Check sheet for the modelled part. Datum: model origin and axes. Units: mm. Face numbers are marked on the shaded views. Give positions to 0.01 mm unless a question says otherwise; leave off trailing zeros. Order: outer loops, then holes, each group sorted by start corner. A loop starts at its lowest first (then second) coordinate and runs counter-clockwise, first axis right, second up.
Item 1: Sectioned sample at C-C on z = -17.5. Record the boundary of the cut face in (x, y).
Item 2: Sectioned sample at A-A on y = 6.5. Record the boundary of the cut face in (x, z).
Item 3: Sectioned sample at D-D on y = 13.75. Record the boundary of the cut face in (x, z), and give its area (3 significant figures).
Item 4: Gauge pin test, flat ends, axial feed: P1, Ø2, axis at x = -5.5, y = 4.5, coming from the +Z side; P2, Ø7.5, axis at y = 8, z = -15, coming from the +X side; P3, Ø0.8, axis at x = -5.5, z = -25.5, coming from the +Y side; P4, Ø4, axis at y = 1.5, z = -20, coming from the -X side. Record the tip position at first contact, or that the pin passes through.
Item 5: Material ranges on line 1 along X through (y, z) = (12, -23.5); line 2 along Y through (x, z) = (-1, -24.25); line 3 along Z through (x, y) = (-8, 4.75), recorded low to high.
Item 6: Sectioned sample at B-B on x = -5.5. Record the boundary of the cut face in (y, z), and give its area (3 significant figures).
Item 7: Release check for a two-part mould opening along Z. For the marked faces 1, 2 and 3 record: released by +Z, released by -Z, zero draft, split by the parting line, or undercut.
Autodesk Inventor part; units mm, degrees
ref_plane "YZ Plane" through (0, 0, 0) normal (1, 0, 0) x (0, 1, 0)
ref_plane "XZ Plane" through (0, 0, 0) normal (0, 1, 0) x (-1, 0, 0)
ref_plane "XY Plane" through (0, 0, 0) normal (0, 0, 1) x (1, 0, 0)
sketch "Sketch2" plane through (0, 0, 0) normal (0, 1, 0) x (-1, 0, 0)
  line L0 (0, 0) -> (0, -26)
  line L1 (0, -26) -> (11, -26)
  line L2 (11, -26) -> (11, 0)
  line L3 (11, 0) -> (0, 0)
  dimension "d2" = 26
  dimension "d3" = 11
extrude "Extrusion1" add sketch "Sketch2" along normal blind 15
sketch "Sketch3" plane through (-11, 0, 0) normal (0, 0, 1) x (1, 0, 0)
  line L0 (0, 0) -> (11, 0)
  line L1 (11, 0) -> (11, 15)
  line L2 (0, 15) -> (11, 15)
  line L3 (0, 0) -> (0, 15)
  line L4 (11, 15) -> (0, 15)
  circle A0 centre (5.5, 15) radius 4.25
  point P0 (9.75, 15)
  point P1 (1.25, 15)
  dimension "d6" = 8.5
extrude "Extrusion2" cut sketch "Sketch3" against normal blind 32.25 contours L2 A0 picked at (4.2044, 14.0026)
sketch "Sketch4" plane through (0, 0, 0) normal (1, 0, 0) x (0, 0, -1)
  line L0 (0, 0) -> (26, 0)
  line L1 (26, 0) -> (26, 15)
  line L2 (0, 15) -> (26, 15)
  line L3 (0, 0) -> (0, 15)
  line L4 (0, 15) -> (4, 15)
  line L5 (0, 15) -> (26, 15)
  line L6 (26, 15) -> (22, 15)
  line L7 (22, 15) -> (22, 12)
  line L8 (0, 10.75) -> (26, 10.75)
  line L9 (22, 12) -> (4, 12)
  line L10 (4, 12) -> (4, 15)
  line L11 (26, 0) -> (0, 0)
  line L12 (13, 0) -> (13, 3)
  arc A0 (4, 12) -> (22, 12) centre (13, 12) ccw
  dimension "d9" = 4
  dimension "d10" = 4
  dimension "d11" = 3
  dimension "d12" = 3
extrude "Extrusion3" cut sketch "Sketch4" against normal blind 32.25 contours A0 L8 | A0 L9 L8 | L2 L7 L9 L10
sketch "Sketch5" plane through (-11, 0, 0) normal (0, 0, 1) x (1, 0, 0)
  arc A0 (1.25, 15) -> (9.75, 15) centre (5.5, 15) ccw
  line L0 (0, 15) -> (1.25, 15)
  line L1 (0, 0) -> (0, 15)
  line L2 (0, 0) -> (11, 0)
  line L3 (11, 0) -> (11, 15)
  line L4 (9.75, 15) -> (11, 15)
  arc A1 (1.25, 15) -> (9.75, 15) centre (5.5, 15) ccw
  line L5 (5.5, 10.75) -> (7, 10.75)
  line L6 (7, 10.75) -> (4, 10.75)
  line L7 (4, 10.75) -> (4.7672, 11.9025)
  line L8 (4.7672, 11.9025) -> (5.5, 11.9025)
  line L9 (5.5, 11.9025) -> (5.5, 10.75)
  line L10 (7, 10.75) -> (6.2328, 11.9025)
  line L11 (6.2328, 11.9025) -> (5.5, 11.9025)
  arc A2 (1.25, 15) -> (9.75, 15) centre (5.5, 15) ccw
  line L12 (11, 15) -> (9.75, 15)
  line L13 (11, 0) -> (11, 15)
  line L14 (11, 0) -> (0, 0)
  line L15 (0, 0) -> (0, 15)
  line L16 (1.25, 15) -> (0, 15)
  line L17 (5.5, 10.75) -> (4, 10.75)
  line L18 (4, 10.75) -> (4.7672, 11.9025)
  line L19 (6.2328, 11.9025) -> (6.1284, 11.9025)
  line L20 (6.2328, 11.9025) -> (4.7672, 11.9025)
  line L21 (6.2328, 11.9025) -> (7, 10.75)
  line L22 (7, 10.75) -> (4, 10.75)
  arc A3 (1.25, 15) -> (9.75, 15) centre (5.5, 15) ccw
  line L23 (11, 15) -> (9.75, 15)
  line L24 (11, 0) -> (11, 15)
  line L25 (11, 0) -> (0, 0)
  line L26 (0, 0) -> (0, 15)
  line L27 (1.25, 15) -> (0, 15)
  arc A4 (1.25, 15) -> (9.75, 15) centre (5.5, 15) ccw
  line L28 (11, 15) -> (9.75, 15)
  line L29 (11, 0) -> (11, 15)
  line L30 (11, 0) -> (0, 0)
  line L31 (0, 0) -> (0, 15)
  line L32 (1.25, 15) -> (0, 15)
  point P0 (4.1472, 10.9711)
  point P1 (6.8528, 10.9711)
  dimension "d15" = 1.5
  dimension "d16" = 3
extrude "Extrusion4" add sketch "Sketch5" against normal blind 1 contours L7 L8 L9 A0 | L9 L11 L10 A0
sketch "Sketch6" plane through (0, 0, -26) normal (0, 0, -1) x (-1, 0, 0)
  arc A0 (1.25, 15) -> (9.75, 15) centre (5.5, 15) ccw
  line L0 (0, 15) -> (1.25, 15)
  line L1 (0, 0) -> (0, 15)
  line L2 (0, 0) -> (11, 0)
  line L3 (11, 0) -> (11, 15)
  line L4 (9.75, 15) -> (11, 15)
  arc A1 (4.1472, 10.9711) -> (6.8528, 10.9711) centre (5.5, 15) ccw
  line L5 (5.5, 10.75) -> (7, 10.75)
  line L6 (4.7672, 11.9025) -> (6.2328, 11.9025)
  line L7 (7, 10.75) -> (6.2328, 11.9025)
  line L8 (6.2328, 11.9025) -> (4.7672, 11.9025)
  line L9 (4.7672, 11.9025) -> (4, 10.75)
  line L10 (4.7672, 11.9025) -> (4.1472, 10.9711)
  line L11 (4, 10.75) -> (5.5, 10.75)
  point P0 (0, 0)
  point P1 (6.8528, 10.9711)
  dimension "d19" = 1.5
extrude "Extrusion5" add sketch "Sketch6" against normal blind 1 contours L9 L6 L7 A0
sketch "Sketch7" plane through (0, 0, 0) normal (0, -1, 0) x (1, 0, 0)
  line L0 (0, -26) -> (-11, -26)
  line L1 (0, 0) -> (0, -26)
  line L2 (-11, 0) -> (0, 0)
  line L3 (-11, -26) -> (-11, 0)
  circle A0 centre (-5.5, -13) radius 5
  dimension "d22" = 10
extrude "Extrusion6" add sketch "Sketch7" along normal blind 2 contours A0
sketch "Sketch8" plane through (-5.5, -2, -13) normal (0, -1, 0) x (1, 0, 0)
  circle A0 centre (0, 0) radius 6
  point P0 (5.5, 13)
  dimension "d25" = 12
extrude "Extrusion7" add sketch "Sketch8" along normal blind 3.5
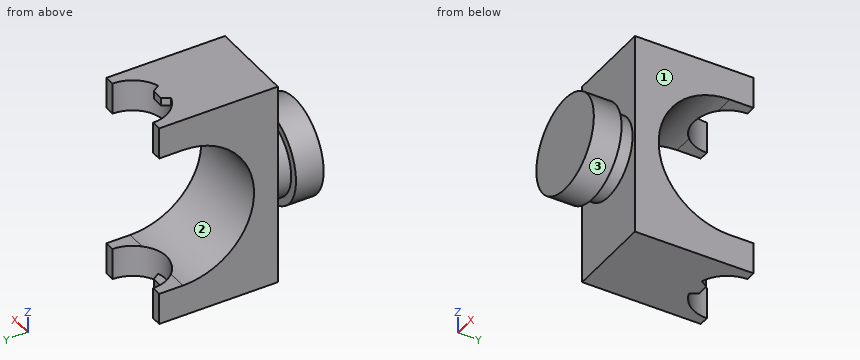
Report:
1. outline: (-11, 0) - (-7.68, 0) - (-7.68, -2) - (-9.47, -2) - (-9.47, -5.5) - (-1.53, -5.5) - (-1.53, -2) - (-3.32, -2) - (-3.32, 0) - (0, 0) - (0, 4.21) - (-11, 4.21) - close
2. outline: (-11, -26) - (0, -26) - (0, -20.12) - (-11, -20.12) - close; (-11, -5.88) - (0, -5.88) - (0, 0) - (-11, 0) - close
3. outline: (-11, -26) - (-9.56, -26) - (-9.56, -22) - (-11, -22) - close; (-11, -4) - (-9.56, -4) - (-9.56, 0) - (-11, 0) - close; (-1.44, -26) - (0, -26) - (0, -22) - (-1.44, -22) - close; (-1.44, -4) - (0, -4) - (0, 0) - (-1.44, 0) - close
3. area: 23.0 mm2
4. P1: stops at z = 0
4. P2: passes through
4. P3: stops at y = 11.9
4. P4: stops at x = -11
5. line 1: x = -11 to -8.51, -2.49 to 0
5. line 2: y = 0 to 15
5. line 3: z = -26 to -18.33, -7.67 to 0
6. outline: (-5.5, -19) - (-2, -19) - (-2, -18) - (0, -18) - (0, -26) - (11.9, -26) - (11.9, -25) - (10.75, -25) - (10.75, -21.91) arc R9 cw to (10.75, -4.09) - (10.75, -1) - (11.9, -1) - (11.9, 0) - (0, 0) - (0, -8) - (-2, -8) - (-2, -7) - (-5.5, -7) - close
6. area: 239 mm2
7. face 1: zero draft
7. face 2: undercut
7. face 3: split by the parting line
